Model file for the job. Use its own axes, mm. Round coordinates to 2 decimals unless told otherwise and drop trailing zeros. Order: outer loops, then holes, each group sorted by start corner. A loop starts at its lowest first (then second) coordinate and runs counter-clockwise, first axis right, second up. Notation, with made-up numbers: (81.25, -2) - (127.25, -2) arc R23 ccw to (127.25, 24) - close; hole circle Ø8 at (-34, 11). An arc over 180 degrees is marked (long way). Use one line per item in the form item = value.
from build123d import *

# Parameters (mm, degrees)
EXTRUDE1_DEPTH          = 1.25
CUT_EXTRUDE3_DEPTH      = 2.25
LPATTERN4_COUNT         = 3
LPATTERN4_PITCH         = 2.54
SKETCH2_W               = 1.752893218
SKETCH2_H               = 0.33
CUT_EXTRUDE1_DEPTH      = 2.27
CUT_EXTRUDE1_DEPTH_BACK = 7.35
SKETCH3_W               = 11
SKETCH3_H               = 0.64
EXTRUDE_THIN1_DEPTH     = 0.32
LPATTERN5_COUNT         = 3
LPATTERN5_PITCH         = 2.54
CHAMFER2_SIZE           = 0.6
CHAMFER2_SIZE2          = 0.105796188
CHAMFER2_PART_2_SIZE    = 0.6
CHAMFER2_PART_2_SIZE2   = 0.105796188
CHAMFER2_PART_3_SIZE    = 0.6
CHAMFER2_PART_3_SIZE2   = 0.105796188
CHAMFER2_PART_4_SIZE    = 0.6
CHAMFER2_PART_4_SIZE2   = 0.105796188
CHAMFER2_PART_5_SIZE    = 0.6
CHAMFER2_PART_5_SIZE2   = 0.105796188
CHAMFER2_PART_6_SIZE    = 0.6
CHAMFER2_PART_6_SIZE2   = 0.105796188
CHAMFER2_PART_7_SIZE    = 0.6
CHAMFER2_PART_7_SIZE2   = 0.105796188
CHAMFER2_PART_8_SIZE    = 0.6
CHAMFER2_PART_8_SIZE2   = 0.105796188
CHAMFER2_PART_9_SIZE    = 0.6
CHAMFER2_PART_9_SIZE2   = 0.105796188
CHAMFER2_PART_10_SIZE   = 0.6
CHAMFER2_PART_10_SIZE2  = 0.105796188
CHAMFER2_PART_11_SIZE   = 0.6
CHAMFER2_PART_11_SIZE2  = 0.105796188
CHAMFER2_PART_12_SIZE   = 0.6
CHAMFER2_PART_12_SIZE2  = 0.105796188
CHAMFER2_PART_13_SIZE   = 0.6
CHAMFER2_PART_13_SIZE2  = 0.105796188
CHAMFER2_PART_14_SIZE   = 0.6
CHAMFER2_PART_14_SIZE2  = 0.105796188
CHAMFER2_PART_15_SIZE   = 0.6
CHAMFER2_PART_15_SIZE2  = 0.105796188
CHAMFER2_PART_16_SIZE   = 0.6
CHAMFER2_PART_16_SIZE2  = 0.105796188
CHAMFER2_PART_17_SIZE   = 0.6
CHAMFER2_PART_17_SIZE2  = 0.105796188
CHAMFER2_PART_18_SIZE   = 0.6
CHAMFER2_PART_18_SIZE2  = 0.105796188
CHAMFER2_PART_19_SIZE   = 0.6
CHAMFER2_PART_19_SIZE2  = 0.105796188
CHAMFER2_PART_20_SIZE   = 0.6
CHAMFER2_PART_20_SIZE2  = 0.105796188
CHAMFER2_PART_21_SIZE   = 0.6
CHAMFER2_PART_21_SIZE2  = 0.105796188
CHAMFER2_PART_22_SIZE   = 0.6
CHAMFER2_PART_22_SIZE2  = 0.105796188
CHAMFER2_PART_23_SIZE   = 0.6
CHAMFER2_PART_23_SIZE2  = 0.105796188
CHAMFER2_PART_24_SIZE   = 0.6
CHAMFER2_PART_24_SIZE2  = 0.105796188


with BuildPart() as part:
    # Sketch1 → Extrude1 (new body, symmetric)
    with BuildSketch(Plane.XY):
        Polygon((-1.27, 0.896446609), (-0.916446609, 1.25), (0.916446609, 1.25), (1.27, 0.896446609), (1.27, -0.896446609), (0.916446609, -1.25), (-0.916446609, -1.25), (-1.27, -0.896446609), align=None)
    extrude1 = extrude(amount=EXTRUDE1_DEPTH, both=True)

    # Sketch4 → Cut-Extrude3 (cut, symmetric)
    with BuildSketch(Plane(origin=(0, 0, 0), x_dir=(1, 0, 0), z_dir=(0, 1, 0))):
        Polygon((-1.27, -1.15), (-1.17, -1.25), (-1.27, -1.25), align=None)
        Polygon((1.17, -1.25), (1.27, -1.15), (1.27, -1.25), align=None)
    cut_extrude3 = extrude(amount=CUT_EXTRUDE3_DEPTH, both=True, mode=Mode.SUBTRACT)

    # LPattern4: Extrude1, Cut-Extrude3 ×3
    with Locations(*[(-i * LPATTERN4_PITCH, 0, 0) for i in range(1, LPATTERN4_COUNT)]):
        add(extrude1)
        add(cut_extrude3, mode=Mode.SUBTRACT)

    # Sketch2 → Cut-Extrude1 (cut, two sides)
    with BuildSketch(Plane(origin=(0, 0, 0), x_dir=(0, -1, 0), z_dir=(1, 0, 0))) as cut_extrude1_sk:
        with Locations((0, 1.085)):
            Rectangle(SKETCH2_W, SKETCH2_H)
    extrude(amount=CUT_EXTRUDE1_DEPTH, mode=Mode.SUBTRACT)
    extrude(cut_extrude1_sk.sketch, amount=-CUT_EXTRUDE1_DEPTH_BACK, mode=Mode.SUBTRACT)

    # Sketch3 → Extrude-Thin1 (add, symmetric)
    with BuildSketch(Plane(origin=(0, 0, 0), x_dir=(0, 0, -1), z_dir=(1, 0, 0))):
        with Locations((-1.75, 0)):
            Rectangle(SKETCH3_W, SKETCH3_H)
    extrude_thin1 = extrude(amount=EXTRUDE_THIN1_DEPTH, both=True)

    # LPattern5: Extrude-Thin1 ×3
    with Locations(*[(-i * LPATTERN5_PITCH, 0, 0) for i in range(1, LPATTERN5_COUNT)]):
        add(extrude_thin1)

    # Chamfer2
    chamfer2_edges = [part.edges().sort_by_distance(p)[0] for p in [
        (0, -0.32, 7.25),
    ]]
    chamfer2_side = [part.faces().sort_by_distance(p)[0] for p in [
        (0, -0.32, 4.25),
    ]]
    chamfer(chamfer2_edges, length=CHAMFER2_SIZE, length2=CHAMFER2_SIZE2, reference=chamfer2_side[0])

    # Chamfer2 part 2
    chamfer2_part_2_edges = [part.edges().sort_by_distance(p)[0] for p in [
        (0, 0.32, -3.75),
    ]]
    chamfer2_part_2_side = [part.faces().sort_by_distance(p)[0] for p in [
        (0, 0.32, -2.335),
    ]]
    chamfer(chamfer2_part_2_edges, length=CHAMFER2_PART_2_SIZE, length2=CHAMFER2_PART_2_SIZE2, reference=chamfer2_part_2_side[0])

    # Chamfer2 part 3
    chamfer2_part_3_edges = [part.edges().sort_by_distance(p)[0] for p in [
        (-0.32, 0, 7.25),
    ]]
    chamfer2_part_3_side = [part.faces().sort_by_distance(p)[0] for p in [
        (-0.32, 0, 4.25),
    ]]
    chamfer(chamfer2_part_3_edges, length=CHAMFER2_PART_3_SIZE, length2=CHAMFER2_PART_3_SIZE2, reference=chamfer2_part_3_side[0])

    # Chamfer2 part 4
    chamfer2_part_4_edges = [part.edges().sort_by_distance(p)[0] for p in [
        (-0.32, 0, -3.75),
    ]]
    chamfer2_part_4_side = [part.faces().sort_by_distance(p)[0] for p in [
        (-0.32, 0, -2.335),
    ]]
    chamfer(chamfer2_part_4_edges, length=CHAMFER2_PART_4_SIZE, length2=CHAMFER2_PART_4_SIZE2, reference=chamfer2_part_4_side[0])

    # Chamfer2 part 5
    chamfer2_part_5_edges = [part.edges().sort_by_distance(p)[0] for p in [
        (0, -0.32, -3.75),
    ]]
    chamfer2_part_5_side = [part.faces().sort_by_distance(p)[0] for p in [
        (0, -0.32, -2.335),
    ]]
    chamfer(chamfer2_part_5_edges, length=CHAMFER2_PART_5_SIZE, length2=CHAMFER2_PART_5_SIZE2, reference=chamfer2_part_5_side[0])

    # Chamfer2 part 6
    chamfer2_part_6_edges = [part.edges().sort_by_distance(p)[0] for p in [
        (0.32, 0, -3.75),
    ]]
    chamfer2_part_6_side = [part.faces().sort_by_distance(p)[0] for p in [
        (0.32, 0, -2.335),
    ]]
    chamfer(chamfer2_part_6_edges, length=CHAMFER2_PART_6_SIZE, length2=CHAMFER2_PART_6_SIZE2, reference=chamfer2_part_6_side[0])

    # Chamfer2 part 7
    chamfer2_part_7_edges = [part.edges().sort_by_distance(p)[0] for p in [
        (0, 0.32, 7.25),
    ]]
    chamfer2_part_7_side = [part.faces().sort_by_distance(p)[0] for p in [
        (0, 0.32, 4.25),
    ]]
    chamfer(chamfer2_part_7_edges, length=CHAMFER2_PART_7_SIZE, length2=CHAMFER2_PART_7_SIZE2, reference=chamfer2_part_7_side[0])

    # Chamfer2 part 8
    chamfer2_part_8_edges = [part.edges().sort_by_distance(p)[0] for p in [
        (0.32, 0, 7.25),
    ]]
    chamfer2_part_8_side = [part.faces().sort_by_distance(p)[0] for p in [
        (0.32, 0, 4.25),
    ]]
    chamfer(chamfer2_part_8_edges, length=CHAMFER2_PART_8_SIZE, length2=CHAMFER2_PART_8_SIZE2, reference=chamfer2_part_8_side[0])

    # Chamfer2 part 9
    chamfer2_part_9_edges = [part.edges().sort_by_distance(p)[0] for p in [
        (-2.54, -0.32, 7.25),
    ]]
    chamfer2_part_9_side = [part.faces().sort_by_distance(p)[0] for p in [
        (-2.54, -0.32, 4.25),
    ]]
    chamfer(chamfer2_part_9_edges, length=CHAMFER2_PART_9_SIZE, length2=CHAMFER2_PART_9_SIZE2, reference=chamfer2_part_9_side[0])

    # Chamfer2 part 10
    chamfer2_part_10_edges = [part.edges().sort_by_distance(p)[0] for p in [
        (-2.54, 0.32, -3.75),
    ]]
    chamfer2_part_10_side = [part.faces().sort_by_distance(p)[0] for p in [
        (-2.54, 0.32, -2.335),
    ]]
    chamfer(chamfer2_part_10_edges, length=CHAMFER2_PART_10_SIZE, length2=CHAMFER2_PART_10_SIZE2, reference=chamfer2_part_10_side[0])

    # Chamfer2 part 11
    chamfer2_part_11_edges = [part.edges().sort_by_distance(p)[0] for p in [
        (-2.86, 0, -3.75),
    ]]
    chamfer2_part_11_side = [part.faces().sort_by_distance(p)[0] for p in [
        (-2.86, 0, -2.335),
    ]]
    chamfer(chamfer2_part_11_edges, length=CHAMFER2_PART_11_SIZE, length2=CHAMFER2_PART_11_SIZE2, reference=chamfer2_part_11_side[0])

    # Chamfer2 part 12
    chamfer2_part_12_edges = [part.edges().sort_by_distance(p)[0] for p in [
        (-2.86, 0, 7.25),
    ]]
    chamfer2_part_12_side = [part.faces().sort_by_distance(p)[0] for p in [
        (-2.86, 0, 4.25),
    ]]
    chamfer(chamfer2_part_12_edges, length=CHAMFER2_PART_12_SIZE, length2=CHAMFER2_PART_12_SIZE2, reference=chamfer2_part_12_side[0])

    # Chamfer2 part 13
    chamfer2_part_13_edges = [part.edges().sort_by_distance(p)[0] for p in [
        (-2.54, -0.32, -3.75),
    ]]
    chamfer2_part_13_side = [part.faces().sort_by_distance(p)[0] for p in [
        (-2.54, -0.32, -2.335),
    ]]
    chamfer(chamfer2_part_13_edges, length=CHAMFER2_PART_13_SIZE, length2=CHAMFER2_PART_13_SIZE2, reference=chamfer2_part_13_side[0])

    # Chamfer2 part 14
    chamfer2_part_14_edges = [part.edges().sort_by_distance(p)[0] for p in [
        (-2.22, 0, -3.75),
    ]]
    chamfer2_part_14_side = [part.faces().sort_by_distance(p)[0] for p in [
        (-2.22, 0, -2.335),
    ]]
    chamfer(chamfer2_part_14_edges, length=CHAMFER2_PART_14_SIZE, length2=CHAMFER2_PART_14_SIZE2, reference=chamfer2_part_14_side[0])

    # Chamfer2 part 15
    chamfer2_part_15_edges = [part.edges().sort_by_distance(p)[0] for p in [
        (-2.54, 0.32, 7.25),
    ]]
    chamfer2_part_15_side = [part.faces().sort_by_distance(p)[0] for p in [
        (-2.54, 0.32, 4.25),
    ]]
    chamfer(chamfer2_part_15_edges, length=CHAMFER2_PART_15_SIZE, length2=CHAMFER2_PART_15_SIZE2, reference=chamfer2_part_15_side[0])

    # Chamfer2 part 16
    chamfer2_part_16_edges = [part.edges().sort_by_distance(p)[0] for p in [
        (-2.22, 0, 7.25),
    ]]
    chamfer2_part_16_side = [part.faces().sort_by_distance(p)[0] for p in [
        (-2.22, 0, 4.25),
    ]]
    chamfer(chamfer2_part_16_edges, length=CHAMFER2_PART_16_SIZE, length2=CHAMFER2_PART_16_SIZE2, reference=chamfer2_part_16_side[0])

    # Chamfer2 part 17
    chamfer2_part_17_edges = [part.edges().sort_by_distance(p)[0] for p in [
        (-5.08, -0.32, 7.25),
    ]]
    chamfer2_part_17_side = [part.faces().sort_by_distance(p)[0] for p in [
        (-5.08, -0.32, 4.25),
    ]]
    chamfer(chamfer2_part_17_edges, length=CHAMFER2_PART_17_SIZE, length2=CHAMFER2_PART_17_SIZE2, reference=chamfer2_part_17_side[0])

    # Chamfer2 part 18
    chamfer2_part_18_edges = [part.edges().sort_by_distance(p)[0] for p in [
        (-5.08, 0.32, -3.75),
    ]]
    chamfer2_part_18_side = [part.faces().sort_by_distance(p)[0] for p in [
        (-5.08, 0.32, -2.335),
    ]]
    chamfer(chamfer2_part_18_edges, length=CHAMFER2_PART_18_SIZE, length2=CHAMFER2_PART_18_SIZE2, reference=chamfer2_part_18_side[0])

    # Chamfer2 part 19
    chamfer2_part_19_edges = [part.edges().sort_by_distance(p)[0] for p in [
        (-5.4, 0, -3.75),
    ]]
    chamfer2_part_19_side = [part.faces().sort_by_distance(p)[0] for p in [
        (-5.4, 0, -2.335),
    ]]
    chamfer(chamfer2_part_19_edges, length=CHAMFER2_PART_19_SIZE, length2=CHAMFER2_PART_19_SIZE2, reference=chamfer2_part_19_side[0])

    # Chamfer2 part 20
    chamfer2_part_20_edges = [part.edges().sort_by_distance(p)[0] for p in [
        (-5.4, 0, 7.25),
    ]]
    chamfer2_part_20_side = [part.faces().sort_by_distance(p)[0] for p in [
        (-5.4, 0, 4.25),
    ]]
    chamfer(chamfer2_part_20_edges, length=CHAMFER2_PART_20_SIZE, length2=CHAMFER2_PART_20_SIZE2, reference=chamfer2_part_20_side[0])

    # Chamfer2 part 21
    chamfer2_part_21_edges = [part.edges().sort_by_distance(p)[0] for p in [
        (-5.08, -0.32, -3.75),
    ]]
    chamfer2_part_21_side = [part.faces().sort_by_distance(p)[0] for p in [
        (-5.08, -0.32, -2.335),
    ]]
    chamfer(chamfer2_part_21_edges, length=CHAMFER2_PART_21_SIZE, length2=CHAMFER2_PART_21_SIZE2, reference=chamfer2_part_21_side[0])

    # Chamfer2 part 22
    chamfer2_part_22_edges = [part.edges().sort_by_distance(p)[0] for p in [
        (-4.76, 0, -3.75),
    ]]
    chamfer2_part_22_side = [part.faces().sort_by_distance(p)[0] for p in [
        (-4.76, 0, -2.335),
    ]]
    chamfer(chamfer2_part_22_edges, length=CHAMFER2_PART_22_SIZE, length2=CHAMFER2_PART_22_SIZE2, reference=chamfer2_part_22_side[0])

    # Chamfer2 part 23
    chamfer2_part_23_edges = [part.edges().sort_by_distance(p)[0] for p in [
        (-5.08, 0.32, 7.25),
    ]]
    chamfer2_part_23_side = [part.faces().sort_by_distance(p)[0] for p in [
        (-5.08, 0.32, 4.25),
    ]]
    chamfer(chamfer2_part_23_edges, length=CHAMFER2_PART_23_SIZE, length2=CHAMFER2_PART_23_SIZE2, reference=chamfer2_part_23_side[0])

    # Chamfer2 part 24
    chamfer2_part_24_edges = [part.edges().sort_by_distance(p)[0] for p in [
        (-4.76, 0, 7.25),
    ]]
    chamfer2_part_24_side = [part.faces().sort_by_distance(p)[0] for p in [
        (-4.76, 0, 4.25),
    ]]
    chamfer(chamfer2_part_24_edges, length=CHAMFER2_PART_24_SIZE, length2=CHAMFER2_PART_24_SIZE2, reference=chamfer2_part_24_side[0])


solid = part.part
(1) Slice it at D-D on z = -0.25. Give the cut face in (x, y), then the cut area to 3 significant figures.
Report:
outline = (-6.35, -0.9) - (-6, -1.25) - (-4.16, -1.25) - (-3.81, -0.9) - (-3.46, -1.25) - (-1.62, -1.25) - (-1.27, -0.9) - (-0.92, -1.25) - (0.92, -1.25) - (1.27, -0.9) - (1.27, 0.9) - (0.92, 1.25) - (-0.92, 1.25) - (-1.27, 0.9) - (-1.62, 1.25) - (-3.46, 1.25) - (-3.81, 0.9) - (-4.16, 1.25) - (-6, 1.25) - (-6.35, 0.9) - close
area = 18.3 mm2
(2) Slice it at A-A on z = 2.25. Give the cut face in (x, y), then the cut area to 3 significant figures.
Report:
outline = (-5.4, -0.32) - (-4.76, -0.32) - (-4.76, 0.32) - (-5.4, 0.32) - close; (-2.86, -0.32) - (-2.22, -0.32) - (-2.22, 0.32) - (-2.86, 0.32) - close; (-0.32, -0.32) - (0.32, -0.32) - (0.32, 0.32) - (-0.32, 0.32) - close
area = 1.23 mm2
(3) Probe probe 1 along X at (y, z) = (-0.2, 4); probe 2 along Z at (x, y) = (-5.5, -0.6); probe 3 along Y at (x, z) = (-5, 4.5). List the from-to ranges inside material, lowest first. Write a range as [from, to].
Report:
probe_1 = [-5.4, -4.76], [-2.86, -2.22], [-0.32, 0.32]
probe_2 = [-0.92, 1.25]
probe_3 = [-0.32, 0.32]
(4) Slice it at C-C on x = -1.75. Give the cut face in (y, z), then the cut area to 3 significant figures.
Report:
outline = (-1.25, -1.25) - (-0.88, -1.25) - (-0.88, -0.92) - (0.88, -0.92) - (0.88, -1.25) - (1.25, -1.25) - (1.25, 1.25) - (-1.25, 1.25) - close
area = 5.67 mm2
(5) Pin check, flat tips, straight feed: pin 1 (1 mm diameter, centred on y = 0.5, z = 4, fed in from -X); pin 2 (0.5 mm diameter, centred on x = 0, z = 5, fed in from -Y); pin 3 (1.5 mm diameter, centred on y = -0.5, z = 5, fed in from +X); pin 4 (1 mm diameter, centred on x = -4.5, y = -0.5, fed in from -Z). Stop position of each tip, or through.
Report:
pin_1 = -5.4
pin_2 = -0.32
pin_3 = 0.32
pin_4 = -3.75
(6) Slice it at B-B on y = 0.5. Give the cut face in (x, z), then the cut area to 3 significant figures.
Report:
outline = (-6.35, -0.92) - (1.27, -0.92) - (1.27, 1.15) - (1.17, 1.25) - (-1.17, 1.25) - (-1.27, 1.15) - (-1.37, 1.25) - (-3.71, 1.25) - (-3.81, 1.15) - (-3.91, 1.25) - (-6.25, 1.25) - (-6.35, 1.15) - close
area = 16.5 mm2
(7) Pull direction Y, two halves, no side cores. Call faces 1 (the face through (-5, 1.25, 0)), 2 (the face through (-1, 0, 1.25)), 3 (the face through (-2, 0, -0.92)): released by +Y, released by -Y, zero draft, split by the parting line, or undercut.
Report:
face_1 = released by +Y
face_2 = zero draft
face_3 = undercut
